Job drawing, mm, ordinate dimensions from the low corner. One solid piece. A direction names the side the tool comes from. Coordinates: 2 decimals unless noted, no trailing zeros. Write each loop counter-clockwise with the first axis right and the second up, starting at its lowest first coordinate (ties: lowest second). Pieces come first, ordered by that corner, then holes.
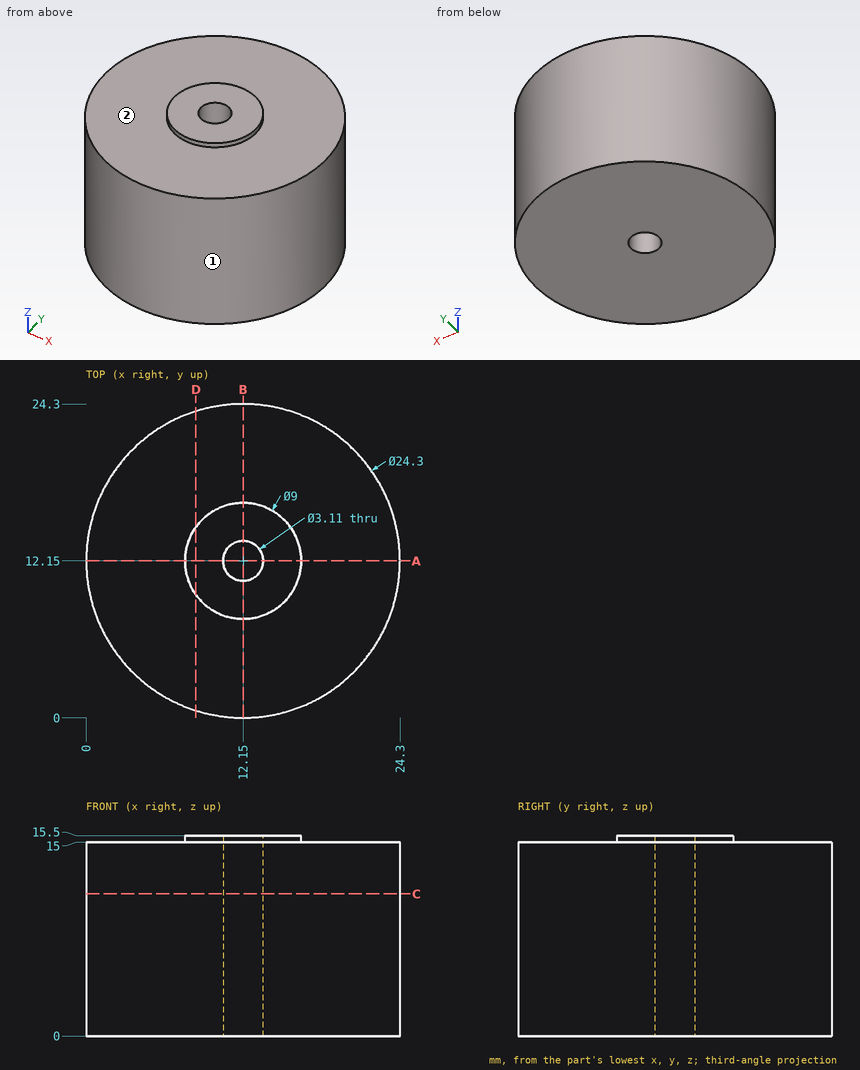
1. Probe line 1 along Y through (x, z) = (12.15, 9) (3 decimals); line 2 along Z through (x, y) = (22.75, 9.5); line 3 along Y through (x, z) = (14.5, 5.5). List the from-to ranges inside material, lowest first.
Computed values:
line 1: y = 0 to 10.595, 13.705 to 24.3
line 2: z = 0 to 15
line 3: y = 0.23 to 24.07
2. Saw through at A-A on y = 12.15. List the corners of the cut face in (x, z) (3 decimals).
Computed values:
outline: (0, 0) - (10.595, 0) - (10.595, 15.5) - (7.65, 15.5) - (7.65, 15) - (0, 15) - close; (13.705, 0) - (24.3, 0) - (24.3, 15) - (16.65, 15) - (16.65, 15.5) - (13.705, 15.5) - close
3. 3-axis set-ups, long thin cutter, end or side, ignore diameter. For the marked faces 1 and 2: which of +Z, -Z, +X, -X, +Y, -Y reach the whole face in a straight line?
Computed values:
face 1: +Z, -Z
face 2: +Z
4. Flat gauge pins, fed straight in: pin 1 (6 mm diameter, centred on y = 3.5, z = 3, fed in from -X); pin 2 (2.5 mm diameter, centred on x = 12.15, y = 12.15, fed in from +Z); pin 3 (1.5 mm diameter, centred on x = 4, z = 11.5, fed in from +Y); pin 4 (8 mm diameter, centred on y = 18, z = 9, fed in from -X). Where does each tip first touch, or does it go through?
Computed values:
pin 1: stops at x = 1.39
pin 2: passes through
pin 3: stops at y = 21.79
pin 4: stops at x = 0.14
5. Saw through at D-D on x = 8.5. List the corners of the cut face in (y, z).
Computed values:
outline: (0.56, 0) - (23.74, 0) - (23.74, 15) - (14.78, 15) - (14.78, 15.5) - (9.52, 15.5) - (9.52, 15) - (0.56, 15) - close
6. Saw through at C-C on z = 11. List the corners of the cut face in (x, y) (3 decimals).
Computed values:
outline: circle Ø24.3 at (12.15, 12.15); hole circle Ø3.11 at (12.15, 12.15)
